Here's how the part is built. I have some questions about the finished solid (model axes, mm). A direction names the side the tool comes from. Give positions to 0.01 mm unless a question says otherwise; leave off trailing zeros. Write each loop counter-clockwise with the first axis right and the second up, starting at its lowest first coordinate (ties: lowest second). Pieces come first, ordered by that corner, then holes. Notation, with made-up numbers: (32.25, 65.5) -> (51.25, 65.5) arc R23 cw to (51.25, 102.5) -> close; hole circle Ø9 at (-35, -11.75). An arc over 180 degrees is marked (long way). Return JSON: item names as keys, results as strings.
Autodesk Inventor part; units mm, degrees
ref_plane "YZ Plane" through (0, 0, 0) normal (1, 0, 0) x (0, 1, 0)
ref_plane "XZ Plane" through (0, 0, 0) normal (0, 1, 0) x (-1, 0, 0)
ref_plane "XY Plane" through (0, 0, 0) normal (0, 0, 1) x (1, 0, 0)
sketch "Sketch1" plane through (0, 0, 0) normal (0, 1, 0) x (-1, 0, 0)
  line L0 (0, -2) -> (0, -28)
  line L1 (2, -30) -> (48, -30)
  line L2 (50, -28) -> (50, -2)
  line L3 (48, 0) -> (2, 0)
  arc A0 (50, -2) -> (48, 0) centre (48, -2) ccw
  arc A1 (48, -30) -> (50, -28) centre (48, -28) ccw
  arc A2 (0, -28) -> (2, -30) centre (2, -28) ccw
  arc A3 (2, 0) -> (0, -2) centre (2, -2) ccw
  point P0 (0, 0)
  point P1 (0, -30)
  point P2 (50, -30)
  point P3 (50, 0)
  dimension "d0" = 30
  dimension "d1" = 50
  dimension "d4" = 2
extrude "Extrusion1" add sketch "Sketch1" along normal blind 2.4
sketch "Sketch2" plane through (0, 2.4, 0) normal (0, 1, 0) x (1, 0, 0)
  line L0 (0, 2) -> (0, 28)
  line L1 (-50, 28) -> (-50, 2)
  line L2 (-50, 17.5) -> (-50, 12.5)
  line L3 (-50, 15) -> (-25, 15)
  line L4 (-25, 15) -> (-40, 15)
  line L5 (-40, 15) -> (-25, 15)
  line L6 (-25, 15) -> (-10, 15)
  circle A0 centre (-40, 15) radius 2.5
  circle A1 centre (-10, 15) radius 2.5
  dimension "d22" = 5
  dimension "d62" = 25
  dimension "d63" = 15
  dimension "d64" = 15
  dimension "d65" = 5
  dimension "d66" = 5
extrude "Extrusion2" cut sketch "Sketch2" against normal blind 2.4
sketch "Sketch3" plane through (0, 2.4, 0) normal (0, 1, 0) x (1, 0, 0)
  line L0 (0, 0) -> (-25, 0)
  line L1 (-48, 0) -> (-2, 0)
  line L2 (-25, 0) -> (-25, 29.9791)
  line L3 (-28, 27.9998) -> (-22, 27.9998) construction
  line L4 (-28, 26.9998) -> (-22, 26.9998)
  line L5 (-22, 28.9998) -> (-28, 28.9998)
  arc A0 (-28, 28.9998) -> (-28, 26.9998) centre (-28, 27.9998) ccw
  arc A1 (-22, 26.9998) -> (-22, 28.9998) centre (-22, 27.9998) ccw
  line L6 (-2, 30) -> (-48, 30)
  line L7 (-27.8848, 2) -> (-21.8848, 2) construction
  line L8 (-27.8848, 1) -> (-21.8848, 1)
  line L9 (-21.8848, 3) -> (-27.8848, 3)
  arc A2 (-27.8848, 3) -> (-27.8848, 1) centre (-27.8848, 2) ccw
  arc A3 (-21.8848, 1) -> (-21.8848, 3) centre (-21.8848, 2) ccw
  point P0 (-25, 27.9998)
  point P1 (-24.8848, 2)
  dimension "d28" = 25
  dimension "d29" = 3
  dimension "d30" = 2
  dimension "d31" = 2.0002
  dimension "d32" = 3
  dimension "d33" = 2
  dimension "d34" = 2
extrude "Extrusion3" cut sketch "Sketch3" along normal mid plane 66
sketch "Sketch5" plane through (0, 2.4, 0) normal (0, 1, 0) x (1, 0, 0)
  line L0 (0, 2) -> (0, 28)
  line L1 (0, 15) -> (-25, 15)
  line L2 (-25, 15) -> (-25, 22)
  circle A0 centre (-25, 22) radius 2
  line L3 (-25, 15) -> (-25, 8)
  circle A1 centre (-25, 8) radius 2
  point P0 (0, 0)
  dimension "d43" = 25
  dimension "d44" = 7
  dimension "d45" = 4
  dimension "d46" = 7
  dimension "d47" = 4
extrude "Extrusion5" cut sketch "Sketch5" against normal blind 66
sketch "Sketch6" plane through (0, 2.4, 0) normal (0, 1, 0) x (1, 0, 0)
  line L0 (0, 2) -> (0, 28)
  line L1 (0, 15) -> (-12.5, 15)
  line L2 (-12.5, 15) -> (-12.5, 22)
  line L3 (-12.5, 22) -> (-12.5, 8)
  circle A0 centre (-12.5, 22) radius 2
  circle A1 centre (-12.5, 8) radius 2
  line L4 (-50.3101, 15) -> (-37.8101, 15)
  line L5 (-37.8101, 15) -> (-37.8101, 22)
  line L6 (-37.8101, 22) -> (-37.8101, 8)
  circle A2 centre (-37.8101, 22) radius 2
  circle A3 centre (-37.8101, 8) radius 2
  point P0 (0, 0)
  dimension "d50" = 12.5
  dimension "d51" = 7
  dimension "d52" = 14
  dimension "d53" = 4
  dimension "d54" = 4
  dimension "d55" = 12.5
  dimension "d56" = 7
  dimension "d57" = 14
  dimension "d58" = 4
  dimension "d59" = 4
extrude "Extrusion6" cut sketch "Sketch6" against normal blind 66
sketch "Sketch7" plane through (0, 2.4, 0) normal (0, 1, 0) x (1, 0, 0)
  line L0 (-48, 0) -> (-2, 0)
  line L1 (-48, 0) -> (-48, 15)
  line L2 (-48, 15) -> (-25, 15)
  circle A0 centre (-25, 15) radius 2
  point P0 (0, 0)
  dimension "d67" = 15
  dimension "d68" = 4
extrude "Extrusion7" cut sketch "Sketch7" against normal through all
properties part number "Cart"
1. Suppose I cut it at A-A, the plane z = -15. List the corners of the cut face in (x, y) for me.
Taken from the geometry:
{"outline": "(-50, 0) -> (-42.5, 0) -> (-42.5, 2.4) -> (-50, 2.4) -> close; (-37.5, 0) -> (-27, 0) -> (-27, 2.4) -> (-37.5, 2.4) -> close; (-23, 0) -> (-12.5, 0) -> (-12.5, 2.4) -> (-23, 2.4) -> close; (-7.5, 0) -> (0, 0) -> (0, 2.4) -> (-7.5, 2.4) -> close"}
2. Suppose I cut it at C-C, the plane y = 0.45. Count the separate pieces of the cut face and the enclosed holes in it, and give its area (3 significant figures).
Taken from the geometry:
{"separate pieces": "1", "enclosed holes": "11", "area": "1,340 mm²"}
3. For pin 1 Ø4.5 at (x, z) = (-10, -15) entering from -Y, with a flat end and sliding along its axis, tell me the tip position at first contact or that it passes through.
Taken from the geometry:
{"pin 1": "passes through"}
4. Suppose I cut it at D-D, the plane x = -25. List the corners of the cut face in (y, z) for me, and give its area (3 significant figures).
Taken from the geometry:
{"outline": "(0, -30) -> (2.4, -30) -> (2.4, -29) -> (0, -29) -> close; (0, -27) -> (2.4, -27) -> (2.4, -24) -> (0, -24) -> close; (0, -20) -> (2.4, -20) -> (2.4, -17) -> (0, -17) -> close; (0, -13) -> (2.4, -13) -> (2.4, -10) -> (0, -10) -> close; (0, -6) -> (2.4, -6) -> (2.4, -3) -> (0, -3) -> close; (0, -1) -> (2.4, -1) -> (2.4, 0) -> (0, 0) -> close", "area": "33.6 mm²"}
5. Suppose I cut it at B-B, the plane x = -10. List the corners of the cut face in (y, z) for me, and give its area (3 significant figures).
Taken from the geometry:
{"outline": "(0, -30) -> (2.4, -30) -> (2.4, -17.5) -> (0, -17.5) -> close; (0, -12.5) -> (2.4, -12.5) -> (2.4, 0) -> (0, 0) -> close", "area": "60.0 mm²"}
6. If we mould it in two halves opening along Z, with no side actions, what happens to faces 1 (the face through (-0.57, 1.18, -0.6)), 2 (the face through (-28.885, 1.183, -1.978)), 3 (the face through (-25, 2.4, -11))? For each: released by +Z, released by -Z, zero draft, split by the parting line, or undercut.
Taken from the geometry:
{"face 1": "released by +Z", "face 2": "undercut", "face 3": "zero draft"}
7. Which directions (+Z, -Z, +X, -X, +Y, -Y) give clear straight access to the entire face, cutting with the end or side of a thin tool? Please do faces 4 (the face through (-25, 0, -11)), 5 (the face through (-25, 1, -29)).
Taken from the geometry:
{"face 4": "+Z, -Z, +X, -X, -Y", "face 5": "+Y, -Y"}
8. If I drill on line 1 (X direction, y = 1.7, z = -22); line 2 (X direction, y = 1.65, z = -15); line 3 (Z direction, x = -25, y = 1.7), over which ranges is the centre line in solid material (lowest first)? Write a range as [from, to].
Taken from the geometry:
{"line 1": "x = [-50, -39.81], [-35.81, -27], [-23, -14.5], [-10.5, 0]", "line 2": "x = [-50, -42.5], [-37.5, -27], [-23, -12.5], [-7.5, 0]", "line 3": "z = [-30, -29], [-27, -24], [-20, -17], [-13, -10], [-6, -3], [-1, 0]"}
